from build123d import *

# Parameters (mm, degrees)
SALIENTE_EXTRUIR1_DEPTH = 0.5


with BuildPart() as part:
    # Croquis1 → Saliente-Extruir1 (new body)
    with BuildSketch(Plane.XY):
        with BuildLine():
            Line((0.499989722, -2.441025539), (0.499989722, -1.936491673))
            ThreePointArc((0.499989722, -1.936491673), (0, 1.999997431), (-0.499989722, -1.936491673))
            Line((-0.499989722, -1.936491673), (-0.499989722, -2.441025539))
            ThreePointArc((-0.499989722, -2.441025539), (-0.999989722, -2.941025539), (-0.499989722, -3.441025539))
            Line((-0.499989722, -3.441025539), (-0.499989722, -3.941025539))
            ThreePointArc((-0.499989722, -3.941025539), (-1.207103771, -3.64812931), (-1.5, -2.941015261))
            ThreePointArc((-1.5, -2.941015261), (-1.584275622, -2.64357108), (-1.786707813, -2.409911864))
            ThreePointArc((-1.786707813, -2.409911864), (0, 3), (1.786707813, -2.409911864))
            ThreePointArc((1.786707813, -2.409911864), (1.576253442, -2.639240432), (1.5, -2.941015261))
            ThreePointArc((1.5, -2.941015261), (1.207103771, -3.64812931), (0.499989722, -3.941025539))
            Line((0.499989722, -3.941025539), (0.499989722, -3.441025539))
            ThreePointArc((0.499989722, -3.441025539), (0.999989722, -2.941025539), (0.499989722, -2.441025539))
        make_face()
    extrude(amount=SALIENTE_EXTRUIR1_DEPTH)


solid = part.part
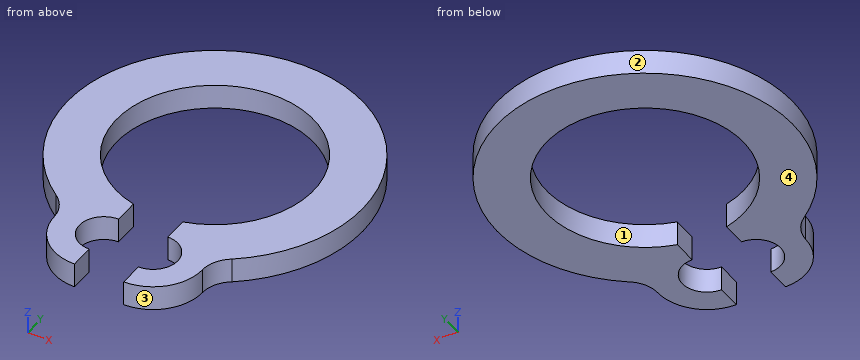
Work out the finished part from the listing and answer in its coordinate system (mm). Face numbers are marked on the shaded views. Coordinates: 2 decimals unless noted, no trailing zeros. Write each loop counter-clockwise with the first axis right and the second up, starting at its lowest first coordinate (ties: lowest second). Pieces come first, ordered by that corner, then holes. Notation, with made-up numbers: M 59,73.25 L 105,73.25 A23 ccw 105,81.25 Z; hole C 42.5,-34 d1. An arc over 180 degrees is marked long. Use one line per item in the form item = value. Start each with the question number.
1. The part is cut by section D-D (x = 0). Give the vertices of the cut face in (y, z).
2. The part is cut by section B-B (z = 0.2). Give the vertices of the cut face in (x, y), plus the area to 3 significant figures.
3. This flat-tipped pin is pushed along its axis until it touches: P1, Ø3, axis at x = 0.5, y = 0.5, coming from the -Z side. Where does it stop, or does it pass through?
4. Straight lines are drawn through the part: probe 1 along X at (y, z) = (0, 0.35); probe 2 along Y at (x, z) = (-0.75, 0.45); probe 3 along X at (y, z) = (1, 0.2). For each, find the intervals that lie inside material, in ascending order. Write a range as from..to.
5. The part is cut by section A-A (y = 0). Give the vertices of the cut face in (x, z), plus the area to 3 significant figures.
6. The mould has two halves that part along Y. Classify the marked faces 1, 2, 3 and 4: released by +Y, released by -Y, zero draft, split by the parting line, or undercut.
7. The part is cut by section C-C (y = -3.25). Give the vertices of the cut face in (x, z), plus the area to 3 significant figures.
Evaluation:
q1.outline = M 2,0 L 3,0 L 3,0.5 L 2,0.5 Z
q2.outline = M -1.79,-2.41 A0.71 cw -1.5,-2.94 A1 ccw -0.5,-3.94 L -0.5,-3.44 A0.5 cw -0.5,-2.44 L -0.5,-1.94 A2 cw long 0.5,-1.94 L 0.5,-2.44 A0.5 cw 0.5,-3.44 L 0.5,-3.94 A1 ccw 1.5,-2.94 A0.64 cw 1.79,-2.41 A3 ccw long Z
q2.area = 15.8 mm^2
q3.P1 = 0
q4.probe_1 = -3..-2, 2..3
q4.probe_2 = -3.91..-3.37, -2.51..-1.85, 1.85..2.9
q4.probe_3 = -2.83..-1.73, 1.73..2.83
q5.outline = M -3,0 L -2,0 L -2,0.5 L -3,0.5 Z; M 2,0 L 3,0 L 3,0.5 L 2,0.5 Z
q5.area = 1.00 mm^2
q6.face_1 = undercut
q6.face_2 = split by the parting line
q6.face_3 = released by -Y
q6.face_4 = zero draft
q7.outline = M -1.45,0 L -0.89,0 L -0.89,0.5 L -1.45,0.5 Z; M 0.89,0 L 1.45,0 L 1.45,0.5 L 0.89,0.5 Z
q7.area = 0.558 mm^2
